```python
from build123d import *

# Parameters (mm, degrees)
SKETCH1_R           = 1.6
BOSS_EXTRUDE1_DEPTH = 5
SKETCH2_W           = 3
SKETCH2_H           = 28.5
BOSS_EXTRUDE2_DEPTH = 10
SKETCH3_W           = 24
SKETCH3_H           = 50
SKETCH3_R           = 1.6
BOSS_EXTRUDE3_DEPTH = 5
BOSS_EXTRUDE4_DEPTH = 3
BOSS_EXTRUDE5_START = -24
BOSS_EXTRUDE5_DEPTH = 3
BOSS_EXTRUDE6_DEPTH = 2.4
FILLET1_R           = 2


with BuildPart() as part:
    # Sketch1 → Boss-Extrude1 (new body)
    with BuildSketch(Plane.XY):
        Polygon((-9, -8.5), (-9, 8.5), (9, 8.5), (9, -8.5), (9, -20), (-9, -20), align=None)
        Circle(SKETCH1_R, mode=Mode.SUBTRACT)
    extrude(amount=BOSS_EXTRUDE1_DEPTH)

    # Sketch2 → Boss-Extrude2 (add)
    with BuildSketch(Plane.XY.offset(5)):
        with Locations((-10.5, -5.75)):
            Rectangle(SKETCH2_W, SKETCH2_H)
        with Locations((10.5, -5.75)):
            Rectangle(SKETCH2_W, SKETCH2_H)
    extrude(amount=-BOSS_EXTRUDE2_DEPTH)

    # Sketch3 → Boss-Extrude3 (add)
    with BuildSketch(Plane(origin=(0, 8.5, 0), x_dir=(1, 0, 0), z_dir=(0, 1, 0))):
        with Locations((0, -30)):
            Rectangle(SKETCH3_W, SKETCH3_H)
        with Locations(Location((0, -45, 0), (0, 0, 270))):
            Circle(SKETCH3_R, mode=Mode.SUBTRACT)
    extrude(amount=-BOSS_EXTRUDE3_DEPTH)

    # Sketch4 → Boss-Extrude4 (add)
    with BuildSketch(Plane.ZY.offset(12)):
        Polygon((28.5, 3.5), (24.257359313, 3.5), (5, -15.757359313), (5, -20), align=None)
    extrude(amount=-BOSS_EXTRUDE4_DEPTH)

    # Sketch4<3> → Boss-Extrude5 (add)
    with BuildSketch(Plane.ZY.offset(12).offset(BOSS_EXTRUDE5_START)):
        Polygon((28.5, 3.5), (24.257359313, 3.5), (5, -15.757359313), (5, -20), align=None)
    extrude(amount=BOSS_EXTRUDE5_DEPTH)

    # Sketch5 → Boss-Extrude6 (add)
    with BuildSketch(Plane.XY.offset(5)):
        Polygon((-5, 3.5), (-5, 2.886751346), (-5, -2.886751346), (0, -5.773502692), (5, -2.886751346), (5, 2.886751346), (5, 3.5), align=None)
        Polygon((3, -1.732050808), (0, -3.464101615), (-3, -1.732050808), (-3, 1.732050808), (0, 3.464101615), (3, 1.732050808), align=None, mode=Mode.SUBTRACT)
    extrude(amount=BOSS_EXTRUDE6_DEPTH)

    # Fillet1
    fillet1_edges = [part.edges().sort_by_distance(p)[0] for p in [
        (-10.5, 3.5, 24.257359313),
        (-10.5, 3.5, 28.5),
        (-10.5, -15.757359313, 5),
        (10.5, -15.757359313, 5),
        (10.5, 3.5, 28.5),
        (10.5, 3.5, 24.257359313),
    ]]
    fillet(fillet1_edges, radius=FILLET1_R)


solid = part.part
```
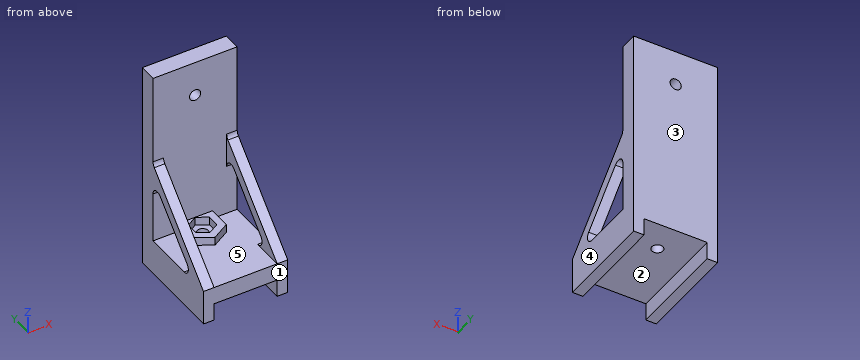
For this review, take the finished solid that the model builds, in its own axes (mm). Face numbers are marked on the shaded views. A direction names the side the tool comes from. Give positions to 0.01 mm unless a question says otherwise; leave off trailing zeros. Write each loop counter-clockwise with the first axis right and the second up, starting at its lowest first coordinate (ties: lowest second). Pieces come first, ordered by that corner, then holes. Notation, with made-up numbers: M -9,67.5 L 40,67.5 A23 ccw 40,96.5 Z; hole C -14,66 d9. An arc over 180 degrees is marked long. One line per item, written item: value.
1) For P1, Ø4, axis at x = -7.5, z = 13.5, coming from the -Y side; P2, Ø0.7, axis at y = 1.5, z = 6, coming from the +X side; P3, Ø1.8, axis at x = 1, y = 0, coming from the +Z side; P4, Ø12, axis at y = -4.5, z = 16, coming from the -X side, all flat-tipped, find the tip position at first contact; note any pin that passes through.
Results are:
P1: stops at y = -12.82
P2: stops at x = 5
P3: stops at z = 5
P4: stops at x = -12
2) Take a section at A-A, the plane y = 6.5. Write out the cut boundary in (x, z).
Results are:
outline: M -12,-5 L -9,-5 L -9,0 L 9,0 L 9,-5 L 12,-5 L 12,55 L -12,55 Z; hole C 0,45 d3.2
3) For line 1 (X direction, y = 3, z = -3); line 2 (Y direction, x = 0, z = 3.45); line 3 (X direction, y = 5.1, z = 45), list the stretches that pass through material, from the lowest coordinate up. Write a range as from..to.
Results are:
line 1: x = -12..-9, 9..12
line 2: y = -20..-1.6, 1.6..8.5
line 3: x = -12..-1.6, 1.6..12
4) Take a section at C-C, the plane y = 1. Write out the cut boundary in (x, z), then the cut area to 3 significant figures.
Results are:
outline: M -12,-5 L -9,-5 L -9,0 L -1.25,0 L -1.25,5 L -3,5 L -3,7.4 L -5,7.4 L -5,5 L -12,5 Z; M -12,21.37 L -9,21.37 L -9,26 L -12,26 Z; M 1.25,0 L 9,0 L 9,-5 L 12,-5 L 12,5 L 5,5 L 5,7.4 L 3,7.4 L 3,5 L 1.25,5 Z; M 9,21.37 L 12,21.37 L 12,26 L 9,26 Z
area: 175 mm²
5) For the marked faces 1 and 2, list the 3-axis set-ups (+Z, -Z, +X, -X, +Y, -Y) from which the entire face can be reached by the end or side of a thin tool; tool diameter is ignored.
Results are:
face 1: +Z, -Z, +X, -X, -Y
face 2: -Z, +Y, -Y
6) Take a section at B-B, the plane z = 45. Write out the cut boundary in (x, y), then the cut area to 3 significant figures.
Results are:
outline: M -12,3.5 L -1.6,3.5 L -1.6,8.5 L -12,8.5 Z; M 1.6,3.5 L 12,3.5 L 12,8.5 L 1.6,8.5 Z
area: 104 mm²
7) The part is to be moulded in two halves that separate along X. For the marked faces 3, 4 and 5, say which applies: +X half, -X half, draft (parallel to the pull), parting line (faces both ways), or undercut.
Results are:
face 3: draft
face 4: +X half
face 5: undercut
8) Take a section at D-D, the plane z = 11.5. Write out the cut boundary in (x, y).
Results are:
outline: M -12,-13.5 L -9,-13.5 L -9,-9.26 L -12,-9.26 Z; M -12,3.5 L 12,3.5 L 12,8.5 L -12,8.5 Z; M 9,-13.5 L 12,-13.5 L 12,-9.26 L 9,-9.26 Z
